Answer from the drawing. Dimensions are ordinates in mm from the lowest x, y and z of the part. A direction names the side the tool comes from. Give positions to 0.01 mm unless a question says otherwise; leave off trailing zeros. Loops run counter-clockwise (first coordinate to the right, second up) from the corner with the lowest first, then second, coordinate; pieces in that order, holes last. Notation, with made-up numbers: (37.25, -9.75) -> (89.25, -9.75) arc R31 ccw to (89.25, 29.25) -> close; hole circle Ø8 at (29, 87.25). An arc over 180 degrees is marked (long way). Return JSON: item names as keys, results as strings. Group by question number.
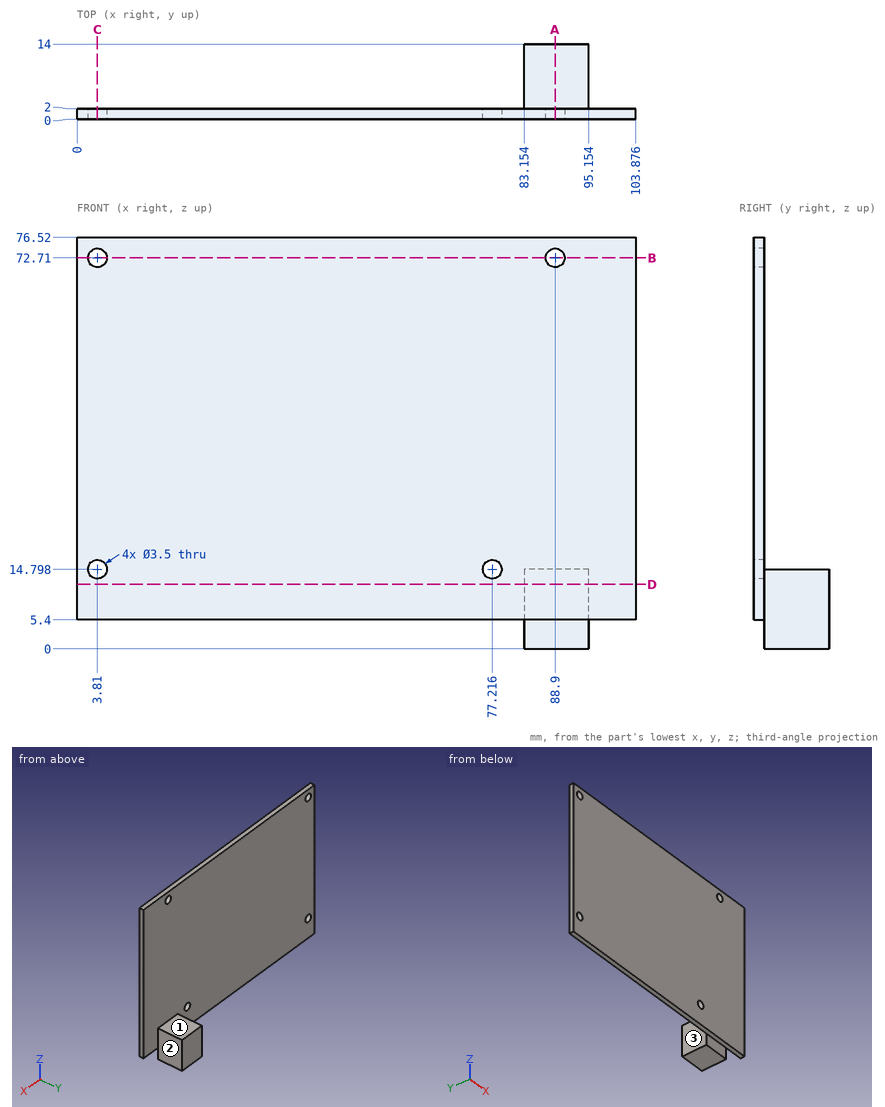
1. Section B-B on z = 72.71 is taken. Determine the outline of the cut face in (x, y), then the cut area to 3 significant figures.
2. Section C-C on x = 3.81 is taken. Determine the outline of the cut face in (y, z), then the cut area to 3 significant figures.
3. Section A-A on x = 88.9 is taken. Determine the outline of the cut face in (y, z), then the cut area to 3 significant figures.
4. Flat-ended cylindrical pins translate along their axes: pin 1 Ø2 at (x, y) = (52.5, 1.5) entering from -Z; pin 2 Ø6 at (y, z) = (7, 6.5) entering from -X; pin 3 Ø6 at (x, z) = (29, 40) entering from +Y. Find the tip coordinate at first contact, or state that the pin passes through.
5. Straight lines are drawn through the part: line 1 (Z direction, x = 3.81, y = 0.7); line 2 (X direction, y = 0.65, z = 72.71); line 3 (Z direction, x = 88.9, y = 1.25). For each, find the intervals that lie inside material, in ascending order. Write a range as from..to.
6. Which of the six approach directions +Z, -Z, +X, -X, +Y, -Y give full straight-line access (tool end or side, diameter ignored) to the marked faces 1, 2 and 3?
7. Section D-D on z = 12 is taken. Determine the outline of the cut face in (x, y).
Completed:
{
 "1": {"outline": "(0, 0) -> (2.06, 0) -> (2.06, 2) -> (0, 2) -> close; (5.56, 0) -> (87.15, 0) -> (87.15, 2) -> (5.56, 2) -> close; (90.65, 0) -> (103.88, 0) -> (103.88, 2) -> (90.65, 2) -> close", "area": "194 mm²"},
 "2": {"outline": "(0, 5.4) -> (2, 5.4) -> (2, 13.05) -> (0, 13.05) -> close; (0, 16.55) -> (2, 16.55) -> (2, 70.96) -> (0, 70.96) -> close; (0, 74.46) -> (2, 74.46) -> (2, 76.52) -> (0, 76.52) -> close", "area": "128 mm²"},
 "3": {"outline": "(0, 5.4) -> (2, 5.4) -> (2, 0) -> (14, 0) -> (14, 14.8) -> (2, 14.8) -> (2, 70.96) -> (0, 70.96) -> close; (0, 74.46) -> (2, 74.46) -> (2, 76.52) -> (0, 76.52) -> close", "area": "313 mm²"},
 "4": {"pin 1": "stops at z = 5.4", "pin 2": "stops at x = 83.15", "pin 3": "stops at y = 2"},
 "5": {"line 1": "z = 5.4..13.05, 16.55..70.96, 74.46..76.52", "line 2": "x = 0..2.06, 5.56..87.15, 90.65..103.88", "line 3": "z = 5.4..70.96, 74.46..76.52"},
 "6": {"face 1": "+Z, +X, -X, +Y", "face 2": "+Z, -Z, +X, +Y", "face 3": "+Z, -Z, -X, +Y"},
 "7": {"outline": "(0, 0) -> (103.88, 0) -> (103.88, 2) -> (95.15, 2) -> (95.15, 14) -> (83.15, 14) -> (83.15, 2) -> (0, 2) -> close"}
}
